Read the model definition and answer for the solid it produces. Units are mm, in the model's axes. Face numbers are marked on the shaded views. A direction names the side the tool comes from. Coordinates: 2 decimals unless noted, no trailing zeros. Order: outer loops, then holes, each group sorted by start corner. A loop starts at its lowest first (then second) coordinate and runs counter-clockwise, first axis right, second up. Notation, with made-up numbers: M 14.5,-38.5 L 37.5,-38.5 A27 cw 37.5,-8.5 Z; hole C 15.5,-33 d9. An arc over 180 degrees is marked long. Use a Markdown table: item, result. Add a question column.
1) Find the intervals of material crossed by probe 1 along Y at (x, z) = (1.5, 9); probe 2 along X at (y, z) = (4, 3.5); probe 3 along X at (y, z) = (-17, 8.5), in increasing order. Write a range as [from, to].
2) The mould has two halves that part along Y. Classify the marked faces 4, 5 and 6: released by +Y, released by -Y, zero draft, split by the parting line, or undercut.
3) Find section B-B on x = -15.5. Write down the section's boundary in (y, z), plus the area to 3 significant figures.
4) Each of these flat-tipped pins is pushed along its axis until it touches: pin 1 Ø2 at (x, z) = (-2, 8) entering from -Y; pin 2 Ø3.5 at (x, y) = (-40.82, 5.77) entering from +Z; pin 3 Ø5 at (y, z) = (-29.5, 3) entering from +X; pin 4 Ø2.5 at (x, y) = (31.75, 29.57) entering from -Z. Where does it stop, or does it pass through?
5) For the marked faces 1, 2 and 3, determine the directions among +Z, -Z, +X, -X, +Y, -Y from which every point of the face is accessible in a straight line to the end or side of a thin tool.
6) Find section A-A on z = 8. Count the separate pieces of the cut face and the enclosed holes in it, plus the area to 3 significant figures.
from build123d import *

# Parameters (mm, degrees)
SKETCH1_R           = 4.05
SKETCH1_R_2         = 1.5
SKETCH1_R_3         = 5.05
BOSS_EXTRUDE1_DEPTH = 10


with BuildPart() as part:
    # Sketch1 → Boss-Extrude1 (new body)
    with BuildSketch(Plane.XY):
        with BuildLine():
            Line((-36.50585994, 38), (23.49414006, 38))
            ThreePointArc((23.49414006, 38), (32.993428927, 36.45634395), (41.515142146, 31.984234067))
            Line((41.515142146, 31.984234067), (76.680353084, 5.562196244))
            ThreePointArc((76.680353084, 5.562196244), (79.334029485, -14.607546806), (59.473059994, -19.012365084))
            Line((59.473059994, -19.012365084), (33.489782569, -4.016722575))
            ThreePointArc((33.489782569, -4.016722575), (26.256281428, -1.021574208), (18.49414006, 0))
            Line((18.49414006, 0), (-31.50585994, 0))
            ThreePointArc((-31.50585994, 0), (-39.73032204, -1.149380887), (-47.324581503, -4.509451788))
            Line((-47.324581503, -4.509451788), (-102.315148598, -38.635060317))
            ThreePointArc((-102.315148598, -38.635060317), (-121.459805376, -36.232350563), (-123.106127076, -17.0078734))
            Line((-123.106127076, -17.0078734), (-53.947129798, 32.409057863))
            ThreePointArc((-53.947129798, 32.409057863), (-45.663596127, 36.56809178), (-36.50585994, 38))
        make_face()
        with Locations((66.99963225, -5.970908883)):
            Circle(SKETCH1_R, mode=Mode.SUBTRACT)
        with Locations((-44.575814379, 29.653127509)):
            Circle(SKETCH1_R_2, mode=Mode.SUBTRACT)
        with Locations((-40.818103787, 5.765583384)):
            Circle(SKETCH1_R_2, mode=Mode.SUBTRACT)
        with Locations((31.754938755, 29.566776323)):
            Circle(SKETCH1_R_2, mode=Mode.SUBTRACT)
        with Locations((27.4947716, 5.867993419)):
            Circle(SKETCH1_R_2, mode=Mode.SUBTRACT)
        with Locations((-100.821311964, -19.473430923)):
            Circle(SKETCH1_R_3, mode=Mode.SUBTRACT)
        with BuildLine():
            Line((-86.793889829, 0.207662569), (-62.735326509, 15.598189533))
            ThreePointArc((-62.735326509, 15.598189533), (-50.276491752, 12.860645223), (-53.014036062, 0.401810467))
            Line((-53.014036062, 0.401810467), (-77.072599382, -14.988716497))
            ThreePointArc((-77.072599382, -14.988716497), (-89.531434139, -12.251172188), (-86.793889829, 0.207662569))
        make_face(mode=Mode.SUBTRACT)
        with BuildLine():
            Line((-23.016668441, 25.777290149), (11.250740888, 25.781094638))
            ThreePointArc((11.250740888, 25.781094638), (19.317386003, 17.716240499), (11.252531864, 9.649595384))
            Line((11.252531864, 9.649595384), (-23.014877464, 9.645790894))
            ThreePointArc((-23.014877464, 9.645790894), (-31.08152258, 17.710645033), (-23.016668441, 25.777290149))
        make_face(mode=Mode.SUBTRACT)
        with BuildLine():
            Line((39.069043687, 17.688629392), (55.302205937, 7.399981644))
            ThreePointArc((55.302205937, 7.399981644), (56.858473261, 0.45660111), (49.915092727, -1.099666214))
            Line((49.915092727, -1.099666214), (33.681930477, 9.188981534))
            ThreePointArc((33.681930477, 9.188981534), (32.125663153, 16.132362067), (39.069043687, 17.688629392))
        make_face(mode=Mode.SUBTRACT)
    extrude(amount=BOSS_EXTRUDE1_DEPTH)


solid = part.part
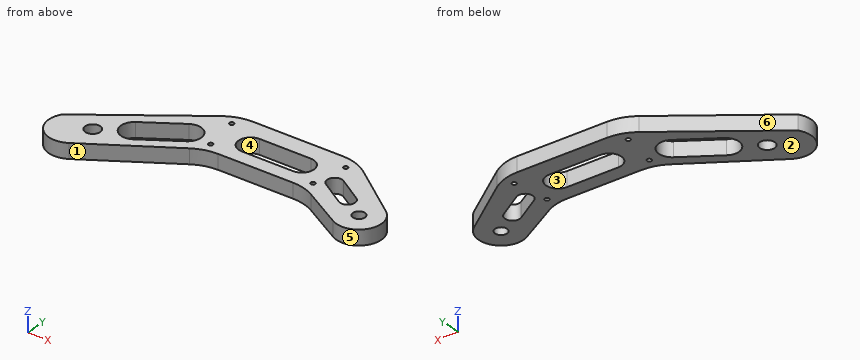
Check result:
| question | item | result |
|---|---|---|
| 1 | probe 1 | y = [0, 9.65], [25.78, 38] |
| 1 | probe 2 | x = [-93.71, -80.87], [-49.79, 41.87], [57.57, 78.28] |
| 1 | probe 3 | x = [-123.1, -105.22], [-96.42, -67.45], [55.99, 77.25] |
| 2 | face 4 | undercut |
| 2 | face 5 | split by the parting line |
| 2 | face 6 | released by +Y |
| 3 | outline | M 0,0 L 9.65,0 L 9.65,10 L 0,10 Z; M 25.78,0 L 38,0 L 38,10 L 25.78,10 Z |
| 3 | area | 219 mm2 |
| 4 | pin 1 | stops at y = 0 |
| 4 | pin 2 | stops at z = 10 |
| 4 | pin 3 | stops at x = -83.57 |
| 4 | pin 4 | passes through |
| 5 | face 1 | +Z, -Z, -Y |
| 5 | face 2 | -Z, +X, -X, +Y, -Y |
| 5 | face 3 | +Z, -Z |
| 6 | separate pieces | 1 |
| 6 | enclosed holes | 9 |
| 6 | area | 5,600 mm2 |
